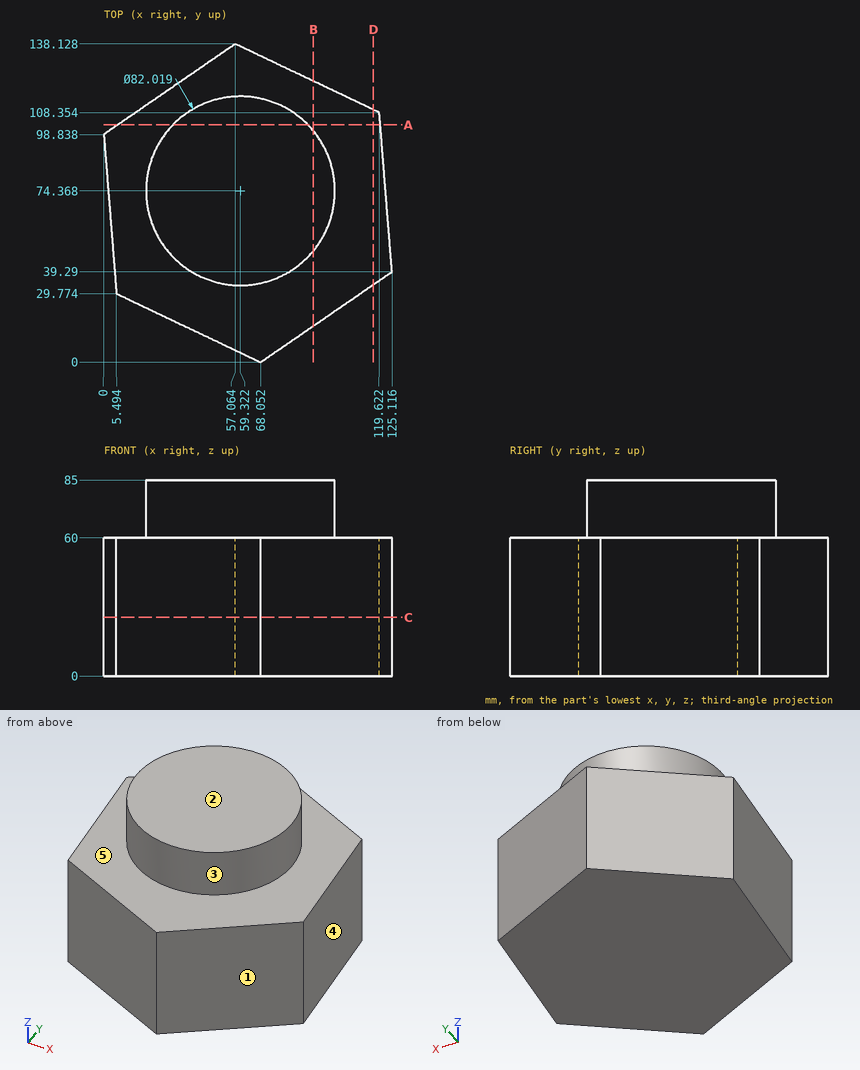
Print and shaded views of the part. All mm, measured from the part's lowest x, y and z. A direction names the side the tool comes from. Give positions to 0.01 mm unless a question says otherwise; leave off trailing zeros. Loops run counter-clockwise (first coordinate to the right, second up) from the corner with the lowest first, then second, coordinate; pieces in that order, holes last.
1) Wall check: line 1 (Z direction, x = 44.5, y = 33); line 2 (X direction, y = 29.5, z = 28) (1 decimal); line 3 (X direction, y = 82.5, z = 31). Give the ranges that are in metal, low to high.
2) Pull direction Y, two halves, no side cores. Call the marked faces 1, 2 and 3: +Y half, -Y half, draft (parallel to the pull), parting line (faces both ways), or undercut.
3) Tool access for the marked faces 4 and 5: list every direction of +Z, -Z, +X, -X, +Y, -Y with a clear straight run to the whole face (end or side of a thin tool).
4) Saw through at C-C (z = 25.5). Write the cut outline in (x, y) (1 decimal), plus the area to 3 significant figures.
5) Saw through at A-A (y = 103). Write the cut outline in (x, z) (1 decimal), plus the area to 3 significant figures.
6) Saw through at D-D (x = 117). Write the cut outline in (y, z).
7) Flat gauge pins, fed straight in: pin 1 Ø12 at (y, z) = (81, 22.5) entering from +X (1 decimal); pin 2 Ø3 at (x, z) = (69, 68) entering from -Y; pin 3 Ø6 at (y, z) = (64, 51) entering from +X; pin 4 Ø8 at (x, y) = (78, 60.5) entering from -Z. Where does each tip first touch, or does it go through?
8) Saw through at B-B (x = 91). Write the cut outline in (y, z), plus the area to 3 significant figures.
Answer block:
1. line 1: z = 0 to 60
1. line 2: x = 6.1 to 110.9
1. line 3: x = 1.3 to 121.68
2. face 1: -Y half
2. face 2: draft
2. face 3: parting line
3. face 4: +Z, -Z, +X, +Y
3. face 5: +Z
4. outline: (0, 98.8) - (5.5, 29.8) - (68.1, 0) - (125.1, 39.3) - (119.6, 108.4) - (57.1, 138.1) - close
4. area: 12,500 mm2
5. outline: (6, 0) - (120, 0) - (120, 60) - (88.7, 60) - (88.7, 85) - (30, 85) - (30, 60) - (6, 60) - close
5. area: 8,310 mm2
6. outline: (33.7, 0) - (109.6, 0) - (109.6, 60) - (33.7, 60) - close
7. pin 1: stops at x = 122.3
7. pin 2: stops at y = 34.18
7. pin 3: stops at x = 123.39
7. pin 4: stops at z = 0
8. outline: (15.8, 0) - (121.98, 0) - (121.98, 60) - (100.41, 60) - (100.41, 85) - (48.32, 85) - (48.32, 60) - (15.8, 60) - close
8. area: 7,670 mm2
